Input: part model. Units: mm. Frame: model coordinates. A direction names the side the tool comes from. Round coordinates to 2 decimals unless told otherwise and drop trailing zeros. Loops run counter-clockwise (first coordinate to the right, second up) from the corner with the lowest first, then second, coordinate; pieces in that order, holes last. Notation, with made-up numbers: (-24, 56.5) -> (4, 56.5) arc R21 cw to (4, 74.5) -> close; hole circle Ø3 at (62.25, 59). An arc over 180 degrees is marked (long way). One line per question, with ' | ' between items. Start each with the question number.
Q1. Access query for faces 1 (the face through (3.76, 6.49, 1.48)), 2 (the face through (3.494, 5.481, 3.542)), 3 (the face through (-2, 2, 4)). Directions: +Z, -Z, +X, -X, +Y, -Y. A direction counts if a zero-diameter tool reaches every point of the face in a straight line with its end or side. Return the directions, or none.
Q2. Cut plane A-A on z = 3.65. Return loops of the section in (x, y).
Q3. Contact query for flat-ended pins moving along their axis: P1, Ø2, axis at x = -1.5, z = 1, coming from the -Y side; P2, Ø1, axis at x = -2, z = 3, coming from the +Y side; P3, Ø1, axis at y = -2, z = 3, coming from the -X side. Output: stop coordinate, or through.
Q4. Material intervals for L1, parallel to Z at x = -5.5, y = -2; L2, parallel to Y at x = -3.75, z = 0.75; L3, parallel to Y at x = 4.75, z = 4.5, sorted ascending.
from build123d import *

# Parameters (mm, degrees)
F1_DEPTH = 3
F2_DEPTH = 4
F3_DEPTH = 5


with BuildPart() as f1:
    # F0 (on Top) → F1 (new body)
    with BuildSketch(Plane.XY):
        with BuildLine():
            ThreePointArc((-4.6512770507, -5.8835042107), (3.2684416868, -6.750354727), (7.5, 0))
            ThreePointArc((7.5, 0), (6.7340096327, 3.3019864123), (4.5925028622, 5.9294955486))
            ThreePointArc((4.5925028622, 5.9294955486), (4.5757009883, 5.9424709057), (4.5588624549, 5.9553986531))
            add(Edge.make_bspline(
                [(5.023105082, 4.1253382086), (4.8092727011, 5.1100586092), (4.527040183, 5.9204651186), (4.5588624549, 5.9553986531)],
                knots=[0.8306208955, 0.8306208955, 0.8306208955, 0.8306208955, 0.9756992936, 0.9756992936, 0.9756992936, 0.9756992936], degree=3))
            ThreePointArc((5.023105082, 4.1253382086), (6.1196479896, 2.1908693443), (6.5, 0))
            ThreePointArc((6.5, 0), (3.0889160794, -5.7191430699), (-3.5641838321, -5.4356778428))
            add(Edge.make_bspline(
                [(-4.6512770507, -5.8835042107), (-4.2900632598, -5.7354905481), (-3.928715743, -5.5872181197), (-3.5641838321, -5.4356778428)],
                knots=[0, 0, 0, 0, 0.0706710697, 0.0706710697, 0.0706710697, 0.0706710697], degree=3))
        make_face()
        with BuildLine():
            ThreePointArc((4.5588624549, 5.9553986531), (4.5757009883, 5.9424709057), (4.5925028622, 5.9294955486))
            add(Edge.make_bspline(
                [(4.5588624549, 5.9553986531), (4.5641927018, 5.9612500381), (4.5783342026, 5.9453444257), (4.5925028622, 5.9294955486)],
                knots=[0.9756992936, 0.9756992936, 0.9756992936, 0.9756992936, 1, 1, 1, 1], degree=3))
        make_face()
        with BuildLine():
            ThreePointArc((-5.0316628164, -5.5616876308), (-4.8441431229, -5.7257556187), (-4.6512770507, -5.8835042107))
            add(Edge.make_bspline(
                [(-4.6512770507, -5.8835042107), (-4.2900632598, -5.7354905481), (-3.928715743, -5.5872181197), (-3.5641838321, -5.4356778428)],
                knots=[0, 0, 0, 0, 0.0706710697, 0.0706710697, 0.0706710697, 0.0706710697], degree=3))
            ThreePointArc((-3.5641838321, -5.4356778428), (-3.9139668667, -5.1894954828), (-4.2468013663, -4.920841204))
            add(Edge.make_bspline(
                [(-5.0316628164, -5.5616876308), (-4.7695889387, -5.3492466161), (-4.5073526376, -5.1366155732), (-4.2468013663, -4.920841204)],
                knots=[0, 0, 0, 0, 0.0643179691, 0.0643179691, 0.0643179691, 0.0643179691], degree=3))
        make_face()
        with BuildLine():
            add(Edge.make_bspline(
                [(5.023105082, 4.1253382086), (4.8092727011, 5.1100586092), (4.527040183, 5.9204651186), (4.5588624549, 5.9553986531)],
                knots=[0.8306208955, 0.8306208955, 0.8306208955, 0.8306208955, 0.9756992936, 0.9756992936, 0.9756992936, 0.9756992936], degree=3))
            ThreePointArc((4.5588624549, 5.9553986531), (3.7441973902, 6.4985372125), (2.8657193097, 6.9309200571))
            ThreePointArc((2.8657193097, 6.9309200571), (2.7819893161, 6.9649504984), (2.6978553142, 6.99796947))
            add(Edge.make_bspline(
                [(2.5499079288, 5.9789605748), (2.5902453757, 6.5226766795), (2.603911247, 6.9348960376), (2.6978553142, 6.99796947)],
                knots=[0.8367623992, 0.8367623992, 0.8367623992, 0.8367623992, 0.947721835, 0.947721835, 0.947721835, 0.947721835], degree=3))
            ThreePointArc((2.5499079288, 5.9789605748), (3.8982830175, 5.2012872941), (5.023105082, 4.1253382086))
        make_face()
        with BuildLine():
            ThreePointArc((2.6978553142, 6.99796947), (-6.3873242431, 3.9309145263), (-5.0316628164, -5.5616876308))
            add(Edge.make_bspline(
                [(-5.0316628164, -5.5616876308), (-4.7695889387, -5.3492466161), (-4.5073526376, -5.1366155732), (-4.2468013663, -4.920841204)],
                knots=[0, 0, 0, 0, 0.0643179691, 0.0643179691, 0.0643179691, 0.0643179691], degree=3))
            ThreePointArc((-4.2468013663, -4.920841204), (-5.5155490696, 3.4392904008), (2.5499079288, 5.9789605748))
            add(Edge.make_bspline(
                [(2.5499079288, 5.9789605748), (2.5902453757, 6.5226766795), (2.603911247, 6.9348960376), (2.6978553142, 6.99796947)],
                knots=[0.8367623992, 0.8367623992, 0.8367623992, 0.8367623992, 0.947721835, 0.947721835, 0.947721835, 0.947721835], degree=3))
        make_face()
        with BuildLine():
            ThreePointArc((2.6978553142, 6.99796947), (2.7819893161, 6.9649504984), (2.8657193097, 6.9309200571))
            add(Edge.make_bspline(
                [(2.6978553142, 6.99796947), (2.7421167455, 7.0276863056), (2.8041982628, 6.9799000242), (2.8657193097, 6.9309200571)],
                knots=[0.947721835, 0.947721835, 0.947721835, 0.947721835, 1, 1, 1, 1], degree=3))
        make_face()
    extrude(amount=F1_DEPTH)

    # F0 (on Top) → F2 (join)
    with BuildSketch(Plane.XY):
        with BuildLine():
            ThreePointArc((2.5499079288, 5.9789605748), (-5.5155490696, 3.4392904008), (-4.2468013663, -4.920841204))
            add(Edge.make_bspline(
                [(-4.2468013663, -4.920841204), (-3.5341805064, -4.3306874282), (-1.8083867278, -2.8177742323), (0.4891946402, 0.4568857751), (2.3494442904, 3.7188761281), (2.5242955811, 5.6337268784), (2.5499079288, 5.9789605748)],
                knots=[0.0643179691, 0.0643179691, 0.0643179691, 0.0643179691, 0.2402308565, 0.4980071555, 0.7663084696, 0.8367623992, 0.8367623992, 0.8367623992, 0.8367623992], degree=3))
        make_face()
        with BuildLine():
            add(Edge.make_bspline(
                [(-3.5641838321, -5.4356778428), (-2.691011307, -5.0726895768), (-0.3985062942, -4.0909828194), (3.8347343504, -1.9210278531), (5.5329932743, 1.2110813852), (5.1336844397, 3.6161087413), (5.023105082, 4.1253382086)],
                knots=[0.0706710697, 0.0706710697, 0.0706710697, 0.0706710697, 0.239951274, 0.5060052495, 0.7555963551, 0.8306208955, 0.8306208955, 0.8306208955, 0.8306208955], degree=3))
            ThreePointArc((-3.5641838321, -5.4356778428), (3.0889160794, -5.7191430699), (6.5, 0))
            ThreePointArc((6.5, 0), (6.1196479896, 2.1908693443), (5.023105082, 4.1253382086))
        make_face()
    extrude(amount=F2_DEPTH)

    # F0 (on Top) → F3 (join)
    with BuildSketch(Plane.XY):
        with BuildLine():
            ThreePointArc((-4.2468013663, -4.920841204), (-3.9139668667, -5.1894954828), (-3.5641838321, -5.4356778428))
            add(Edge.make_bspline(
                [(-3.5641838321, -5.4356778428), (-2.691011307, -5.0726895768), (-0.3985062942, -4.0909828194), (3.8347343504, -1.9210278531), (5.5329932743, 1.2110813852), (5.1336844397, 3.6161087413), (5.023105082, 4.1253382086)],
                knots=[0.0706710697, 0.0706710697, 0.0706710697, 0.0706710697, 0.239951274, 0.5060052495, 0.7555963551, 0.8306208955, 0.8306208955, 0.8306208955, 0.8306208955], degree=3))
            ThreePointArc((5.023105082, 4.1253382086), (3.8982830175, 5.2012872941), (2.5499079288, 5.9789605748))
            add(Edge.make_bspline(
                [(-4.2468013663, -4.920841204), (-3.5341805064, -4.3306874282), (-1.8083867278, -2.8177742323), (0.4891946402, 0.4568857751), (2.3494442904, 3.7188761281), (2.5242955811, 5.6337268784), (2.5499079288, 5.9789605748)],
                knots=[0.0643179691, 0.0643179691, 0.0643179691, 0.0643179691, 0.2402308565, 0.4980071555, 0.7663084696, 0.8367623992, 0.8367623992, 0.8367623992, 0.8367623992], degree=3))
        make_face()
    extrude(amount=F3_DEPTH)


solid = f1.part
Results:
1) face 1: +Z, -Z, +X, +Y | face 2: +Z | face 3: +Z, -X, +Y
2) outline: circle Ø13 at (0, 0)
3) P1: y = -7.48 | P2: y = 7.35 | P3: x = -7.35
4) L1: 0 to 4 | L2: -6.5 to 6.5 | L3: 0.11 to 4.44
